Check sheet for the modelled part. Datum: model origin and axes. Units: mm. A direction names the side the tool comes from. Give positions to 0.01 mm unless a question says otherwise; leave off trailing zeros. Use CSV: the item, a comma, the result in double quotes.
from build123d import *

# Parameters (mm, degrees)
BOSS_EXTRUDE1_DEPTH     = 2
SKETCH2_R               = 1.375
CUT_EXTRUDE1_DEPTH      = 2
CUT_EXTRUDE5_DEPTH      = 10
CUT_EXTRUDE3_DEPTH      = 46.516465277
CUT_EXTRUDE3_DEPTH_BACK = 46.516465277
SKETCH12_R              = 1.375


with BuildPart() as part:
    # Sketch1 → Boss-Extrude1 (new body)
    with BuildSketch(Plane(origin=(0, 0, 0), x_dir=(1, 0, 0), z_dir=(0, 1, 0))):
        with BuildLine():
            Line((-6.5, 0), (6.5, 0))
            Line((6.5, 0), (6.5, 5.19))
            add(Edge.make_bspline(
                [(-6.5, 5.19), (0, 3.63), (6.5, 5.19)],
                knots=[0, 0, 0, 1, 1, 1], degree=2))
            Line((-6.5, 5.19), (-6.5, 0))
        make_face()
    extrude(amount=BOSS_EXTRUDE1_DEPTH)

    # Sketch2 → Cut-Extrude1 (cut)
    with BuildSketch(Plane(origin=(0, 2, 0), x_dir=(1, 0, 0), z_dir=(0, 1, 0))):
        with Locations(Location((-4, 2.595, 0), (0, 0, 270))):
            Circle(SKETCH2_R)
        with Locations(Location((4, 2.595, 0), (0, 0, 270))):
            Circle(SKETCH2_R)
    extrude(amount=-CUT_EXTRUDE1_DEPTH, mode=Mode.SUBTRACT)

    # Sketch4 → Loft2 section 0
    with BuildSketch(Plane(origin=(0, 2, 0), x_dir=(1, 0, 0), z_dir=(0, 1, 0))):
        with BuildLine():
            Line((-1.875, 3.75), (1.875, 3.75))
            Line((1.875, 3.75), (1.875, 0))
            Line((1.875, 0), (-1.875, 0))
            Line((-1.875, 0), (-1.875, 3.75))
        make_face()
    # Sketch6 → Loft2 section 1
    with BuildSketch(Plane(origin=(0, 44.75, 0), x_dir=(1, 0, 0), z_dir=(0, 1, 0))):
        with BuildLine():
            Line((-6, 1), (6, 1))
            Line((6, 1), (6, -2.75))
            Line((6, -2.75), (-6, -2.75))
            Line((-6, -2.75), (-6, 1))
        make_face()
    loft()

    # Sketch16 → Cut-Extrude5 (cut)
    with BuildSketch(Plane(origin=(0, 0.248475921, -3.86267114), x_dir=(-1, 0, 0), z_dir=(0, 0.06419480263840949, -0.9979373864698206))):
        Polygon((-1.875, 1.755144263), (-1.875, 34.593503242), (-6, 44.593503242), align=None)
        Polygon((1.875, 34.593503242), (1.875, 1.755144263), (6, 44.593503242), align=None)
    extrude(amount=-CUT_EXTRUDE5_DEPTH, mode=Mode.SUBTRACT)

    # Sketch12 → Cut-Extrude3 (cut, two sides: drawn at the far end of the back side and taken through both)
    with BuildSketch(Plane.XY.offset(-CUT_EXTRUDE3_DEPTH_BACK)):
        with Locations(Location((-2.5, 41.75, 0), (0, 0, 90))):
            Circle(SKETCH12_R)
        with Locations(Location((2.5, 41.75, 0), (0, 0, 90))):
            Circle(SKETCH12_R)
    extrude(amount=CUT_EXTRUDE3_DEPTH + CUT_EXTRUDE3_DEPTH_BACK, mode=Mode.SUBTRACT)


solid = part.part
1. Scan lines: line 1 along Y through (x, z) = (-5.25, -3.25); line 2 along X through (y, z) = (41.75, 0.4) (3 decimals); line 3 along Y through (x, z) = (5.25, -0.5). Record each from-to range of solid material in increasing order.
Completed:
line 1,"y = 0 to 2"
line 2,"x = -4.802 to -3.875, -1.125 to 1.125, 3.875 to 4.802"
line 3,"y = 0 to 2, 42.9 to 44.75"
2. Sectioned sample at A-A, the plane z = -3.25. State how many separate pieces and enclosed holes the cut face has, and give its area (3 significant figures).
Completed:
separate pieces,"3"
enclosed holes,"0"
area,"45.5 mm²"
3. Set-up check for faces 4 (the face through (0, 0, -3)), 5 (the face through (0, 2, -4)): record each of +Z, -Z, +X, -X, +Y, -Y from which the full face is reachable in a straight line by a thin tool's end or side.
Completed:
face 4,"+Z, -Z, +X, -X, -Y"
face 5,"-Z"
4. Release check for a two-part mould opening along Z. For faces 1 (the face through (0, 1, 0)), 2 (the face through (-2.56, 40.376, 0.655)), 3 (the face through (-4.527, 1.014, -1.325)) record: released by +Z, released by -Z, zero draft, split by the parting line, or undercut.
Completed:
face 1,"released by +Z"
face 2,"zero draft"
face 3,"undercut"
5. Go/stop test with flat-tipped pins: pin 1 Ø4.5 at (y, z) = (13, -0.5) entering from -X (3 decimals); pin 2 Ø2 at (x, y) = (1.5, 26) entering from -Z; pin 3 Ø1 at (x, y) = (-0.5, 1.5) entering from +Z. Record where each tip stops, or that it passes through.
Completed:
pin 1,"stops at x = -1.875"
pin 2,"stops at z = -2.27"
pin 3,"stops at z = 0"
